For this review, take the finished solid that the model builds, in its own axes (mm). A direction names the side the tool comes from. Give positions to 0.01 mm unless a question says otherwise; leave off trailing zeros. Write each loop counter-clockwise with the first axis right and the second up, starting at its lowest first coordinate (ties: lowest second). Pieces come first, ordered by that corner, then holes. Notation, with made-up numbers: M 35.25,53 L 48.25,53 A32 cw 48.25,86 Z; hole C -3.75,19 d1. An arc over 180 degrees is marked long. One line per item, written item: value. Start each with the question number.
Item 1: Consider section D-D, the plane y = 8. Write out the cut boundary in (x, z), and give its area (3 significant figures).
Item 2: Clearance check with a flat-ended pin moving along its axis: pin 1 Ø13.5 at (x, z) = (-20, -20) entering from +Y. State where the tip first meets the part, or that it passes through.
Item 3: To check wall thickness, follow probe 1 along X at (y, z) = (7, -20); probe 2 along Z at (x, y) = (0, 8); probe 3 along Z at (x, y) = (-21.5, 5). State the ranges of each line that lie inside material, in increasing order.
Item 4: Tool access review of faces 4 (the face through (25.1, 7.6, -25.5)), 5 (the face through (23.04, 1.52, -23.32)): name each direction out of +Z, -Z, +X, -X, +Y, -Y from which nothing blocks a thin tool from reaching the whole face with its end or side.
Item 5: Consider section C-C, the plane z = 20. Write out the cut boundary in (x, y), and give its area (3 significant figures).
Item 6: Consider section A-A, the plane z = 0. Write out the cut boundary in (x, y), and give its area (3 significant figures).
Item 7: Mouldability with a two-part tool opening along Y and no side actions: class faces 1 (the face through (-1, 12, -9)), 2 (the face through (8, 0, -1)), 3 (the face through (23.04, 1.52, 16.68)) as released by +Y, released by -Y, zero draft, split by the parting line, or undercut.
Item 8: Consider section B-B, the plane x = 20. Write out the cut boundary in (y, z).
```python
from build123d import *

# Parameters (mm, degrees)
SKETCH_1_W             = 80
SKETCH_1_H             = 80
EXTRUDE_1_DEPTH        = 12
HOLE_WIZARD_M141_D     = 12
HOLE_WIZARD_M141_DEPTH = 12
SKETCH_12_R            = 4.5
CUT_EXTRUDE_1_DEPTH    = 13
SKETCH_13_R            = 7.5
CUT_EXTRUDE_2_DEPTH    = 9


with BuildPart() as part:
    # Эскиз1 → Бобышка-Вытянуть1 (new body)
    with BuildSketch(Plane(origin=(0, 0, 0), x_dir=(1, 0, 0), z_dir=(0, 1, 0))):
        Rectangle(SKETCH_1_W, SKETCH_1_H)
    extrude(amount=EXTRUDE_1_DEPTH)

    # Отверстие обработанное метчиком M141
    with Locations(Plane(origin=(0, 12, 0), x_dir=(1, 0, 0), z_dir=(0, 1, 0))):
        with Locations((0, 0)):
            Hole(HOLE_WIZARD_M141_D / 2, depth=HOLE_WIZARD_M141_DEPTH)

    # Эскиз12 → Вырез-Вытянуть1 (cut, through all)
    with BuildSketch(Plane(origin=(0, 12, 0), x_dir=(1, 0, 0), z_dir=(0, 1, 0))):
        with Locations(Location((-20, 20, 0), (0, 0, 270))):  # turned: the seam where the file's is
            Circle(SKETCH_12_R)
        with Locations(Location((20, 20, 0), (0, 0, 270))):  # turned: the seam where the file's is
            Circle(SKETCH_12_R)
        with Locations(Location((20, -20, 0), (0, 0, 270))):  # turned: the seam where the file's is
            Circle(SKETCH_12_R)
        with Locations(Location((-20, -20, 0), (0, 0, 270))):  # turned: the seam where the file's is
            Circle(SKETCH_12_R)
    extrude(amount=-CUT_EXTRUDE_1_DEPTH, mode=Mode.SUBTRACT)

    # Эскиз13 → Вырез-Вытянуть2 (cut)
    with BuildSketch(Plane(origin=(0, 12, 0), x_dir=(1, 0, 0), z_dir=(0, 1, 0))):
        with Locations(Location((-20, 20, 0), (0, 0, 270))):  # turned: the seam where the file's is
            Circle(SKETCH_13_R)
        with Locations(Location((20, 20, 0), (0, 0, 270))):  # turned: the seam where the file's is
            Circle(SKETCH_13_R)
        with Locations(Location((20, -20, 0), (0, 0, 270))):  # turned: the seam where the file's is
            Circle(SKETCH_13_R)
        with Locations(Location((-20, -20, 0), (0, 0, 270))):  # turned: the seam where the file's is
            Circle(SKETCH_13_R)
    extrude(amount=-CUT_EXTRUDE_2_DEPTH, mode=Mode.SUBTRACT)


solid = part.part
```
Model answer:
1. outline: M -40,-40 L 40,-40 L 40,40 L -40,40 Z; hole C -20,-20 d15; hole C -20,20 d15; hole C 0,0 d12; hole C 20,-20 d15; hole C 20,20 d15
1. area: 5,580 mm2
2. pin 1: stops at y = 3
3. probe 1: x = -40 to -27.5, -12.5 to 12.5, 27.5 to 40
3. probe 2: z = -40 to -6, 6 to 40
3. probe 3: z = -40 to -27.35, -12.65 to 12.65, 27.35 to 40
4. face 4: +Y
4. face 5: +Y, -Y
5. outline: M -40,0 L -24.5,0 L -24.5,3 L -27.5,3 L -27.5,12 L -40,12 Z; M -15.5,0 L 15.5,0 L 15.5,3 L 12.5,3 L 12.5,12 L -12.5,12 L -12.5,3 L -15.5,3 Z; M 24.5,0 L 40,0 L 40,12 L 27.5,12 L 27.5,3 L 24.5,3 Z
5. area: 636 mm2
6. outline: M -40,0 L -6,0 L -6,12 L -40,12 Z; M 6,0 L 40,0 L 40,12 L 6,12 Z
6. area: 816 mm2
7. face 1: released by +Y
7. face 2: released by -Y
7. face 3: zero draft
8. outline: M 0,-40 L 12,-40 L 12,-27.5 L 3,-27.5 L 3,-24.5 L 0,-24.5 Z; M 0,-15.5 L 3,-15.5 L 3,-12.5 L 12,-12.5 L 12,12.5 L 3,12.5 L 3,15.5 L 0,15.5 Z; M 0,24.5 L 3,24.5 L 3,27.5 L 12,27.5 L 12,40 L 0,40 Z
